from build123d import *

# Parameters (mm, degrees)
EXTRUDE_1_DEPTH     = 2
SKETCH_2_R          = 1.7
CUT_EXTRUDE_1_DEPTH = 2
SKETCH_3_R          = 1.7
CUT_EXTRUDE_2_DEPTH = 3
SKETCH_4_RX         = 15
SKETCH_4_RY         = 6
CUT_EXTRUDE_3_DEPTH = 3
FILLET_1_R          = 5
FILLET_2_R          = 10
CUT_EXTRUDE_5_DEPTH = 3


with BuildPart() as part:
    # 草图1 → 凸台-拉伸1 (new body)
    with BuildSketch(Plane(origin=(0, 0, 0), x_dir=(1, 0, 0), z_dir=(0, 1, 0))):
        Polygon((-10.5, -40), (25.5, -40), (67.5, -40), (67.5, -20), (67.5, 20), (67.5, 40), (25.5, 40), (-10.5, 40), (-67.5, 40), (-67.5, 20), (-67.5, -20), (-67.5, -40), align=None)
    extrude(amount=EXTRUDE_1_DEPTH)

    # 草图2 → 切除-拉伸1 (cut)
    with BuildSketch(Plane(origin=(0, 2, 0), x_dir=(1, 0, 0), z_dir=(0, 1, 0))):
        with Locations(Location((-63.5, 35, 0), (0, 0, 270))):
            Circle(SKETCH_2_R)
        with Locations(Location((63.5, 35, 0), (0, 0, 90))):
            Circle(SKETCH_2_R)
        with Locations(Location((63.5, -35, 0), (0, 0, 270))):
            Circle(SKETCH_2_R)
        with Locations(Location((-63.5, -35, 0), (0, 0, 90))):
            Circle(SKETCH_2_R)
    extrude(amount=-CUT_EXTRUDE_1_DEPTH, mode=Mode.SUBTRACT)

    # 草图3 → 切除-拉伸2 (cut)
    with BuildSketch(Plane(origin=(0, 2, 0), x_dir=(1, 0, 0), z_dir=(0, 1, 0))):
        with Locations(Location((-31, 25, 0), (0, 0, 270))):
            Circle(SKETCH_3_R)
        with Locations(Location((31, 25, 0), (0, 0, 270))):
            Circle(SKETCH_3_R)
        with Locations(Location((-31, -25, 0), (0, 0, 270))):
            Circle(SKETCH_3_R)
        with Locations(Location((31, -25, 0), (0, 0, 270))):
            Circle(SKETCH_3_R)
    extrude(amount=-CUT_EXTRUDE_2_DEPTH, mode=Mode.SUBTRACT)

    # 草图4 → 切除-拉伸3 (cut)
    with BuildSketch(Plane(origin=(0, 2, 0), x_dir=(1, 0, 0), z_dir=(0, 1, 0))):
        with Locations(Location((-39.5, 0), (0, 0, -90))):
            Ellipse(SKETCH_4_RX, SKETCH_4_RY)
        with Locations(Location((39.5, 0), (0, 0, -90))):
            Ellipse(SKETCH_4_RX, SKETCH_4_RY)
        with BuildLine():
            Line((-67.5, 17), (-67.5, -17))
            ThreePointArc((-67.5, -17), (-50.5, 0), (-67.5, 17))
        make_face()
        with BuildLine():
            Line((67.5, 17), (67.5, -17))
            ThreePointArc((67.5, -17), (50.5, 0), (67.5, 17))
        make_face()
        with BuildLine():
            Line((-20, 40), (20, 40))
            ThreePointArc((20, 40), (0, 20), (-20, 40))
        make_face()
        with BuildLine():
            Line((-20, -40), (20, -40))
            ThreePointArc((20, -40), (0, -20), (-20, -40))
        make_face()
    extrude(amount=-CUT_EXTRUDE_3_DEPTH, mode=Mode.SUBTRACT)

    # 圆角1
    fillet_1_edges = [part.edges().sort_by_distance(p)[0] for p in [
        (67.5, 1, -40),
        (67.5, 1, 40),
        (-67.5, 1, 40),
        (-67.5, 1, -40),
    ]]
    fillet(fillet_1_edges, radius=FILLET_1_R)

    # 圆角2
    fillet_2_edges = [part.edges().sort_by_distance(p)[0] for p in [
        (20, 1, -40),
        (-20, 1, -40),
        (-20, 1, 40),
        (20, 1, 40),
        (67.5, 1, 17),
        (67.5, 1, -17),
        (-67.5, 1, -17),
        (-67.5, 1, 17),
    ]]
    fillet(fillet_2_edges, radius=FILLET_2_R)

    # 草图6 → 切除-拉伸5 (cut)
    with BuildSketch(Plane.XZ):
        Polygon((-24.505396053, -12.076400213), (-20.097950719, 12.076400213), (-6.523019093, 12.076400213), (-7.216611088, 8.275516079), (-17.277185706, 8.275516079), (-18.787316377, 0), (-12.246898397, 0), (-12.865682091, -3.390934644), (-18.787316377, -3.390934644), (-20.37225535, -12.076400213), align=None)
        Polygon((14.28012288, 12.076400213), (4.76004096, -12.076400213), (23.095013546, -12.076400213), align=None)
    extrude(amount=-CUT_EXTRUDE_5_DEPTH, mode=Mode.SUBTRACT)


solid = part.part
Model file for the job. Use its own axes, mm. A direction names the side the tool comes from. Give positions to 0.01 mm unless a question says otherwise; leave off trailing zeros. Write each loop counter-clockwise with the first axis right and the second up, starting at its lowest first coordinate (ties: lowest second). Pieces come first, ordered by that corner, then holes. Notation, with made-up numbers: M -9,77 L -5,77 A9 cw -5,86 Z; hole C -10.75,22 d10. An arc over 180 degrees is marked long. One line per item, written item: value. Start each with the question number.
Q1. 3-axis set-ups, long thin cutter, end or side, ignore diameter. For faces 1 (the cylindrical face through (65.73, 0.99, -19.4)), 2 (the flat face through (-1, 0, -1)), 3 (the flat face through (9.6, 1, 0.2)), 4 (the cylindrical face through (-65.73, 0.99, -19.4)): which of +Z, -Z, +X, -X, +Y, -Y reach the whole face in a straight line?
Q2. Saw through at C-C, the plane z = 30.5. Write the cut outline in (x, y).
Q3. Drop flat-ended pins along their axis: pin 1 Ø0.6 at (x, y) = (-13, 1.5) entering from +Z; pin 2 Ø1 at (x, y) = (0.5, 0.5) entering from -Z (3 decimals); pin 3 Ø2 at (x, z) = (-63.5, 35) entering from +Y; pin 4 Ø0.6 at (x, y) = (-14.5, 1) entering from -Z. Give the stop position or say it passes through.
Q4. Saw through at B-B, the plane x = 56. Write the cut outline in (y, z), plus the area to 3 significant figures.
Q5. Saw through at A-A, the plane x = 31. Write the cut outline in (y, z).
Q6. Probe probe 1 along X at (y, z) = (1.5, 10); probe 2 along X at (y, z) = (0.85, -35); probe 3 along X at (y, z) = (0.7, 0.5). List the from-to ranges inside material, lowest first. Write a range as [from, to].
Q7. Two-plate mould, pull along Z, no slides. Class faces 5 (the cylindrical face through (-66.07, 1.01, -38.5)), 6 (the flat face through (18.75, 0.99, -0.17)), 7 (the cylindrical face through (22.581, 0.986, 38.214)): +Z half, -Z half, draft (parallel to the pull), parting line (faces both ways), or undercut.
Q8. Saw through at D-D, the plane y = 0.9. State how many separate pieces and enclosed holes the cut face has, plus the area to 3 significant figures.
Output values:
1. face 1: +X, +Y, -Y
1. face 2: +Z, -Z, +X, -X, -Y
1. face 3: +Y, -Y
1. face 4: -X, +Y, -Y
2. outline: M -67.5,0 L -17.6,0 L -17.6,2 L -67.5,2 Z; M 17.6,0 L 67.5,0 L 67.5,2 L 17.6,2 Z
3. pin 1: stops at z = 25.06
3. pin 2: stops at z = -20.025
3. pin 3: passes through
3. pin 4: stops at z = -26.55
4. outline: M 0,-40 L 2,-40 L 2,-12.52 L 0,-12.52 Z; M 0,12.52 L 2,12.52 L 2,40 L 0,40 Z
4. area: 110 mm²
5. outline: M 0,-40 L 2,-40 L 2,-26.7 L 0,-26.7 Z; M 0,-23.3 L 2,-23.3 L 2,23.3 L 0,23.3 Z; M 0,26.7 L 2,26.7 L 2,40 L 0,40 Z
6. probe 1: x = [-53.75, -43.97], [-35.03, -20.48], [-6.9, 13.46], [15.04, 35.03], [43.97, 53.75]
6. probe 2: x = [-67.5, -65.2], [-61.8, -19.62], [19.62, 61.8], [65.2, 67.5]
6. probe 3: x = [-50.51, -45.5], [-33.5, -22.21], [-18.7, 9.72], [18.51, 33.5], [45.5, 50.51]
7. face 5: -Z half
7. face 6: undercut
7. face 7: +Z half
8. separate pieces: 1
8. enclosed holes: 12
8. area: 7,510 mm²
